For this review, take the finished solid that the model builds, in its own axes (mm). Give positions to 0.01 mm unless a question says otherwise; leave off trailing zeros. Order: outer loops, then holes, each group sorted by start corner. A loop starts at its lowest first (then second) coordinate and runs counter-clockwise, first axis right, second up. Notation, with made-up numbers: M 50,58 L 109,58 A20 ccw 109,71 Z; hole C -7,74 d9. An arc over 180 degrees is marked long. Use CSV: the item, a comma, the result in double quotes. Start each with the question number.
(1) Wall thickness on L1, parallel to Y at x = 0, z = 0.5; L2, parallel to Y at x = -30.5, z = 1.5; L3, parallel to X at y = -33, z = -11.25: over which ranges is each line inside the solid? List them lowest first. Write a range as from..to.
(2) Clearance check with flat-ended pins moving along their axes: P1, Ø1.5, axis at y = -66.5, z = 2.5, coming from the +X side; P2, Ø5, axis at y = -34.5, z = 3.5, coming from the -X side; P3, Ø1.5, axis at y = 38.5, z = 9.5, coming from the +X side. State where each tip first meets the part, or that it passes through.
(3) Consider section A-A (x = 0). Write out the cut boundary in (y, z), and give its area (3 significant figures).
(4) Draft analysis for pull direction Y (two halves, no side actions). For faces 1 (the face through (-13.8, -62.145, 10.319)), 2 (the face through (-13.8, -62.145, -10.319)), 3 (the face through (-20, -64, -12.7)), 4 (the face through (-18.748, -84.427, -12.577)), state which applies: pulls with the +Y half, pulls with the -Y half, needs draft (parallel to the pull), parting line crosses it, or undercut.
(5) Consider section C-C (z = 5.5). Write out the cut boundary in (x, y).
```python
from build123d import *

# Parameters (mm, degrees)
F0_R     = 88.9
F0_R_2   = 63.5
F1_DEPTH = 12.7
F2_SIZE  = 2.54


with BuildPart() as f1:
    # F0 (on Top) → F1 (new body)
    with BuildSketch(Plane.XY):
        Circle(F0_R)
        Circle(F0_R_2, mode=Mode.SUBTRACT)
    extrude(amount=F1_DEPTH)

    # F2
    f2_edges = [f1.edges().sort_by_distance(p)[0] for p in [
        (-88.9, 0, 12.7),
        (-63.5, 0, 12.7),
    ]]
    chamfer(f2_edges, length=F2_SIZE)

    # F3: F1 across face


with BuildPart() as f1_1:
    add(f1.part)
    add(f1.part.mirror(Plane(origin=(0, 0, 0), x_dir=(1, 0, 0), z_dir=(0, 0, -1))))


solid = f1_1.part
```
Check result:
1,L1,"y = -88.9..-63.5, 63.5..88.9"
1,L2,"y = -83.5..-55.7, 55.7..83.5"
1,L3,"x = -81.37..-55.52, 55.52..81.37"
2,P1,"stops at x = 59.83"
2,P2,"stops at x = -82.94"
2,P3,"stops at x = 80.49"
3,outline,"M -88.9,-10.16 L -86.36,-12.7 L -66.04,-12.7 L -63.5,-10.16 L -63.5,10.16 L -66.04,12.7 L -86.36,12.7 L -88.9,10.16 Z; M 63.5,-10.16 L 66.04,-12.7 L 86.36,-12.7 L 88.9,-10.16 L 88.9,10.16 L 86.36,12.7 L 66.04,12.7 L 63.5,10.16 Z"
3,area,"1,260 mm^2"
4,face 1,"undercut"
4,face 2,"undercut"
4,face 3,"needs draft"
4,face 4,"parting line crosses it"
5,outline,"C 0,0 d177.8; hole C 0,0 d127"
